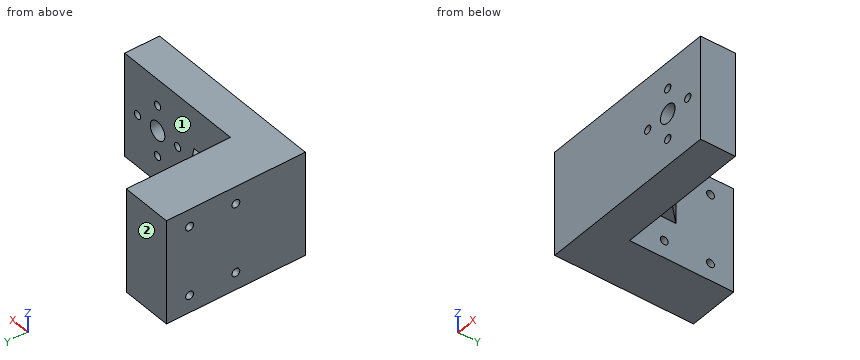
```python
from build123d import *

# Parameters (mm, degrees)
BOSS_EXTRUDE3_DEPTH      = 22.5
BOSS_EXTRUDE3_DEPTH_BACK = 22.5
SKETCH1_W                = 22
SKETCH1_H                = 60
BOSS_EXTRUDE4_DEPTH      = 22.5
BOSS_EXTRUDE4_DEPTH_BACK = 22.5
SKETCH2_W                = 80
SKETCH2_H                = 15
CUT_EXTRUDE1_DEPTH       = 103.5
CUT_EXTRUDE1_DEPTH_BACK  = 103.5
SKETCH3_R                = 4
SKETCH3_R_2              = 1.7
CUT_EXTRUDE2_DEPTH       = 103.5
CUT_EXTRUDE2_DEPTH_BACK  = 103.5
SKETCH4_R                = 1.7
BOSS_EXTRUDE5_DEPTH      = 5
BOSS_EXTRUDE5_DEPTH_BACK = 5


with BuildPart() as part:
    # Sketch1 → Boss-Extrude3 (new, two sides: drawn at the far end of the back side and taken through both)
    with BuildSketch(Plane.XY.offset(-BOSS_EXTRUDE3_DEPTH_BACK)):
        with Locations((11, 30)):
            Rectangle(SKETCH1_W, SKETCH1_H)
    extrude(amount=BOSS_EXTRUDE3_DEPTH + BOSS_EXTRUDE3_DEPTH_BACK)

    # Sketch2 → Boss-Extrude4 (add, two sides: drawn at the far end of the back side and taken through both)
    with BuildSketch(Plane.XY.offset(-BOSS_EXTRUDE4_DEPTH_BACK)):
        with Locations((40, 7.5)):
            Rectangle(SKETCH2_W, SKETCH2_H)
    extrude(amount=BOSS_EXTRUDE4_DEPTH + BOSS_EXTRUDE4_DEPTH_BACK)

    # Sketch3 → Cut-Extrude1 (cut, two sides: drawn at the far end of the back side and taken through both)
    with BuildSketch(Plane(origin=(0, 0, 0), x_dir=(1, 0, 0), z_dir=(0, 1, 0)).offset(-CUT_EXTRUDE1_DEPTH_BACK)):
        with Locations(Location((62, 0, 0), (0, 0, 270))):
            Circle(SKETCH3_R)
        with Locations(Location((73, 0, 0), (0, 0, 270))):
            Circle(SKETCH3_R_2)
        with Locations(Location((51, 0, 0), (0, 0, 270))):
            Circle(SKETCH3_R_2)
        with Locations(Location((62, 11, 0), (0, 0, 270))):
            Circle(SKETCH3_R_2)
        with Locations(Location((62, -11, 0), (0, 0, 270))):
            Circle(SKETCH3_R_2)
    extrude(amount=CUT_EXTRUDE1_DEPTH + CUT_EXTRUDE1_DEPTH_BACK, mode=Mode.SUBTRACT)

    # Sketch4 → Cut-Extrude2 (cut, two sides: drawn at the far end of the back side and taken through both)
    with BuildSketch(Plane(origin=(0, 0, 0), x_dir=(0, 0, -1), z_dir=(1, 0, 0)).offset(-CUT_EXTRUDE2_DEPTH_BACK)):
        with Locations((15, 30)):
            Circle(SKETCH4_R)
        with Locations((-15, 30)):
            Circle(SKETCH4_R)
        with Locations((15, 50)):
            Circle(SKETCH4_R)
        with Locations((-15, 50)):
            Circle(SKETCH4_R)
    extrude(amount=CUT_EXTRUDE2_DEPTH + CUT_EXTRUDE2_DEPTH_BACK, mode=Mode.SUBTRACT)

    # Sketch5 → Boss-Extrude5 (add, two sides: drawn at the far end of the back side and taken through both)
    with BuildSketch(Plane.XY.offset(-BOSS_EXTRUDE5_DEPTH_BACK)):
        Polygon((22, 15), (42, 15), (22, 35), align=None)
    extrude(amount=BOSS_EXTRUDE5_DEPTH + BOSS_EXTRUDE5_DEPTH_BACK)


solid = part.part
```
Can you work these out from the model? Positions are in its coordinate system, mm. Face numbers are marked on the shaded views. A direction names the side the tool comes from. Coordinates: 2 decimals unless noted, no trailing zeros. Order: outer loops, then holes, each group sorted by start corner. A loop starts at its lowest first (then second) coordinate and runs counter-clockwise, first axis right, second up.
1. For the marked faces 1 and 2, which set-ups out of +Z, -Z, +X, -X, +Y, -Y let a thin tool reach every point of the face, with its end or its side?
2. I need wall thicknesses on line 1 (Y direction, x = 4, z = 15); line 2 (X direction, y = 11.5, z = 0); line 3 (Z direction, x = 11, y = 30). Which ranges of each line are inside material? Lowest first, please.
3. I'm going to push flat-ended pins straight in: pin 1 (13 mm diameter, centred on x = 62, z = 0, fed in from -Y); pin 2 (4.5 mm diameter, centred on x = 73, z = 0, fed in from +Y); pin 3 (2 mm diameter, centred on x = 26, z = -0.5, fed in from +Y); pin 4 (4 mm diameter, centred on y = 30, z = 15, fed in from +X). Where does each tip first touch, or does it pass through?
4. If we section it at C-C (z = -11): Please give me the cut outline in (x, y), then the cut area to 3 significant figures.
5. If we section it at A-A (y = 50): Please give me the cut outline in (x, z), then the cut area to 3 significant figures.
6. If we section it at B-B (x = 62): Please give me the cut outline in (y, z).
7. If we section it at D-D (z = 0): Please give me the cut outline in (x, y).
Entries:
1. face 1: +X, +Y
1. face 2: +Z, -Z, +X, -X, +Y
2. line 1: y = 0 to 28.3, 31.7 to 48.3, 51.7 to 60
2. line 2: x = 0 to 49.3, 52.7 to 58, 66 to 71.3, 74.7 to 80
2. line 3: z = -22.5 to -16.7, -13.3 to 13.3, 16.7 to 22.5
3. pin 1: stops at y = 0
3. pin 2: stops at y = 15
3. pin 3: stops at y = 32
3. pin 4: stops at x = 22
4. outline: (0, 0) - (60.3, 0) - (60.3, 15) - (22, 15) - (22, 60) - (0, 60) - close; (63.7, 0) - (80, 0) - (80, 15) - (63.7, 15) - close
4. area: 2,140 mm2
5. outline: (0, -22.5) - (22, -22.5) - (22, -16.7) - (0, -16.7) - close; (0, -13.3) - (22, -13.3) - (22, 13.3) - (0, 13.3) - close; (0, 16.7) - (22, 16.7) - (22, 22.5) - (0, 22.5) - close
5. area: 840 mm2
6. outline: (0, -22.5) - (15, -22.5) - (15, -12.7) - (0, -12.7) - close; (0, -9.3) - (15, -9.3) - (15, -4) - (0, -4) - close; (0, 4) - (15, 4) - (15, 9.3) - (0, 9.3) - close; (0, 12.7) - (15, 12.7) - (15, 22.5) - (0, 22.5) - close
7. outline: (0, 0) - (49.3, 0) - (49.3, 15) - (42, 15) - (22, 35) - (22, 60) - (0, 60) - close; (52.7, 0) - (58, 0) - (58, 15) - (52.7, 15) - close; (66, 0) - (71.3, 0) - (71.3, 15) - (66, 15) - close; (74.7, 0) - (80, 0) - (80, 15) - (74.7, 15) - close
